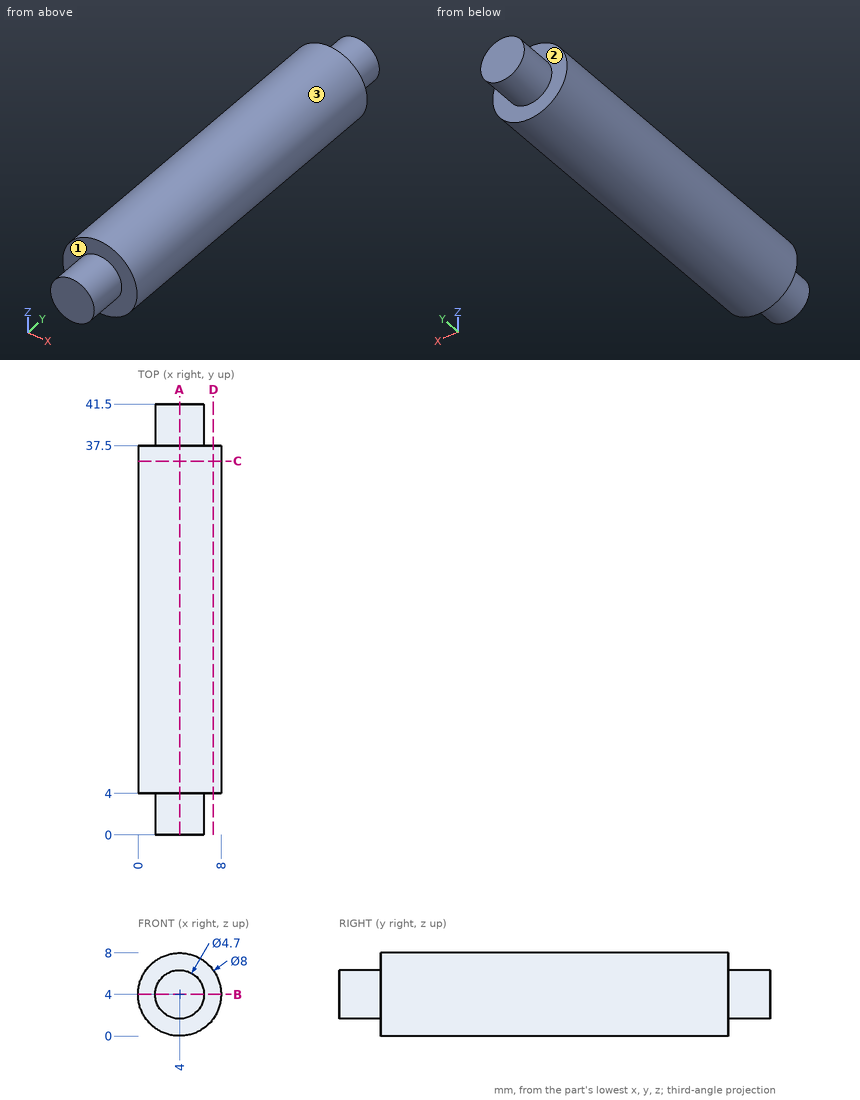
Part print with two shaded views. Sizes in mm from the minimum x, y, z corner. A direction names the side the tool comes from. Give positions to 0.01 mm unless a question says otherwise; leave off trailing zeros. Order: outer loops, then holes, each group sorted by start corner. A loop starts at its lowest first (then second) coordinate and runs counter-clockwise, first axis right, second up.
(1) Saw through at D-D, the plane x = 7.25. Give the cut face in (y, z), then the cut area to 3 significant figures.
(2) Saw through at B-B, the plane z = 4. Give the cut face in (x, y).
(3) Tool access for the marked faces 1, 2 and 3: list every direction of +Z, -Z, +X, -X, +Y, -Y with a clear straight run to the whole face (end or side of a thin tool).
(4) Saw through at C-C, the plane y = 36. Give the cut face in (x, z), then the cut area to 3 significant figures.
(5) Saw through at A-A, the plane x = 4. Give the cut face in (y, z), then the cut area to 3 significant figures.
(6) Flat gauge pins, fed straight in: pin 1 (4 mm diameter, centred on x = 1.5, y = 18.5, fed in from +Z); pin 2 (2 mm diameter, centred on x = 1.5, y = 4.5, fed in from +Z). Where does each tip first touch, or does it go through?
(7) Drill centre lines: L1, parallel to Y at x = 0.5, z = 5; L2, parallel to Z at x = 3.75, y = 37; L3, parallel to X at y = 9.5, z = 4.5. Where is each one in solid material? Low to high.
Results found:
1. outline: (4, 1.67) - (37.5, 1.67) - (37.5, 6.33) - (4, 6.33) - close
1. area: 156 mm2
2. outline: (0, 4) - (1.65, 4) - (1.65, 0) - (6.35, 0) - (6.35, 4) - (8, 4) - (8, 37.5) - (6.35, 37.5) - (6.35, 41.5) - (1.65, 41.5) - (1.65, 37.5) - (0, 37.5) - close
3. face 1: -Y
3. face 2: +Y
3. face 3: +Y, -Y
4. outline: circle Ø8 at (4, 4)
4. area: 50.3 mm2
5. outline: (0, 1.65) - (4, 1.65) - (4, 0) - (37.5, 0) - (37.5, 1.65) - (41.5, 1.65) - (41.5, 6.35) - (37.5, 6.35) - (37.5, 8) - (4, 8) - (4, 6.35) - (0, 6.35) - close
5. area: 306 mm2
6. pin 1: stops at z = 7.97
6. pin 2: stops at z = 7.71
7. L1: y = 4 to 37.5
7. L2: z = 0.01 to 7.99
7. L3: x = 0.03 to 7.97
